The model under review builds one solid part; all positions refer to its coordinate system, in mm. A direction names the side the tool comes from. Coordinates: 2 decimals unless noted, no trailing zeros. Order: outer loops, then holes, each group sorted by start corner. A loop starts at its lowest first (then second) coordinate and runs counter-clockwise, first axis right, second up. Notation, with made-up numbers: (2.5, 48.25) - (15.5, 48.25) arc R17 ccw to (15.5, 62.25) - close; hole circle Ø7 at (-31, -4.75). An arc over 180 degrees is marked (long way). Answer in a Markdown table with one row per item.
```python
from build123d import *

# Parameters (mm, degrees)
SKETCH1_W           = 50
SKETCH1_H           = 55
BOSS_EXTRUDE1_DEPTH = 2
SKETCH2_W           = 5.3
SKETCH2_H           = 4
SKETCH2_R           = 1.5
SKETCH2_W_2         = 10.5
SKETCH2_H_2         = 4.678571429
CUT_EXTRUDE1_DEPTH  = 10


with BuildPart() as part:
    # Sketch1 → Boss-Extrude1 (new body)
    with BuildSketch(Plane(origin=(0, 0, 0), x_dir=(0, 0, -1), z_dir=(1, 0, 0))):
        Rectangle(SKETCH1_W, SKETCH1_H)
    extrude(amount=BOSS_EXTRUDE1_DEPTH)

    # Sketch2 → Cut-Extrude1 (cut)
    with BuildSketch(Plane(origin=(2, 0, 0), x_dir=(0, 0, -1), z_dir=(1, 0, 0))):
        with Locations((-2.284317843, -4.476763319)):
            Rectangle(SKETCH2_W, SKETCH2_H)
        with Locations((2.25, -3.75)):
            Circle(SKETCH2_R)
        Polygon((5.25, 6.75), (5.25, 2.071428571), (5.5, 2.071428571), (5.5, 7.071428571), (-5.5, 7.071428571), (-5.5, 2.071428571), (-5.25, 2.071428571), (-5.25, 6.75), align=None)
        with Locations((0, 4.410714286)):
            Rectangle(SKETCH2_W_2, SKETCH2_H_2)
    extrude(amount=-CUT_EXTRUDE1_DEPTH, mode=Mode.SUBTRACT)


solid = part.part
```
Item 1: We need section D-D, the plane y = -3.75. Write out the cut boundary in (x, z).
Check values:
| item | result |
|---|---|
| outline | (0, -25) - (2, -25) - (2, -3.75) - (0, -3.75) - close; (0, -0.75) - (2, -0.75) - (2, -0.37) - (0, -0.37) - close; (0, 4.93) - (2, 4.93) - (2, 25) - (0, 25) - close |
Item 2: Tool access review of faces 4 (the face through (1, 7.071, 0)), 5 (the face through (1, -27.5, 0)): name each direction out of +Z, -Z, +X, -X, +Y, -Y from which nothing blocks a thin tool from reaching the whole face with its end or side.
Check values:
| item | result |
|---|---|
| face 4 | +X, -X |
| face 5 | +Z, -Z, +X, -X, -Y |
Item 3: To check wall thickness, follow line 1 (Y direction, x = 1.25, z = -2.25); line 2 (Z direction, x = 1, y = -3); line 3 (Z direction, x = 1.15, y = -5). State the ranges of each line that lie inside material, in increasing order. Write a range as from..to.
Check values:
| item | result |
|---|---|
| line 1 | -27.5..-5.25, -2.25..2.07, 7.07..27.5 |
| line 2 | -25..-3.55, -0.95..-0.37, 4.93..25 |
| line 3 | -25..-3.08, -1.42..-0.37, 4.93..25 |
Item 4: Mouldability with a two-part tool opening along Z and no side actions: class faces 1 (the face through (1, -5, 4.934)), 2 (the face through (0, 0, 0)), 3 (the face through (1, 0, 25)) as +Z half, -Z half, draft (parallel to the pull), parting line (faces both ways), or undercut.
Check values:
| item | result |
|---|---|
| face 1 | undercut |
| face 2 | draft |
| face 3 | +Z half |
Item 5: We need section B-B, the plane z = -2.25. Write out the cut boundary in (x, y), then the cut area to 3 significant figures.
Check values:
| item | result |
|---|---|
| outline | (0, -27.5) - (2, -27.5) - (2, -5.25) - (0, -5.25) - close; (0, -2.25) - (2, -2.25) - (2, 2.07) - (0, 2.07) - close; (0, 7.07) - (2, 7.07) - (2, 27.5) - (0, 27.5) - close |
| area | 94.0 mm^2 |
Item 6: We need section A-A, the plane y = 3. Write out the cut boundary in (x, z).
Check values:
| item | result |
|---|---|
| outline | (0, -25) - (2, -25) - (2, -5.5) - (0, -5.5) - close; (0, 5.5) - (2, 5.5) - (2, 25) - (0, 25) - close |
Item 7: Clearance check with a flat-ended pin moving along its axis: pin 1 Ø3 at (y, z) = (-5, -19) entering from -X. State where the tip first meets the part, or that it passes through.
Check values:
| item | result |
|---|---|
| pin 1 | x = 0 |
Item 8: We need section C-C, the plane x = 1.5. Write out the cut boundary in (y, z), then the cut area to 3 significant figures.
Check values:
| item | result |
|---|---|
| outline | (-27.5, -25) - (27.5, -25) - (27.5, 25) - (-27.5, 25) - close; hole (-6.48, -0.37) - (-2.48, -0.37) - (-2.48, 4.93) - (-6.48, 4.93) - close; hole circle Ø3 at (-3.75, -2.25); hole (2.07, -5.5) - (7.07, -5.5) - (7.07, 5.5) - (2.07, 5.5) - close |
| area | 2,670 mm^2 |
